Geometry check sheet. Reference: drawing and pictorial views, mm from the part's lowest x, y, z. Coordinates: 2 decimals unless noted, no trailing zeros. Write each loop counter-clockwise with the first axis right and the second up, starting at its lowest first coordinate (ties: lowest second). Pieces come first, ordered by that corner, then holes. Notation, with made-up numbers: (20.25, 89.5) - (72.25, 89.5) arc R24 ccw to (72.25, 103.5) - close; hole circle Ø1 at (8, 87). An arc over 180 degrees is marked (long way). Answer as a JSON object with one key per item and string values. Group by question number.
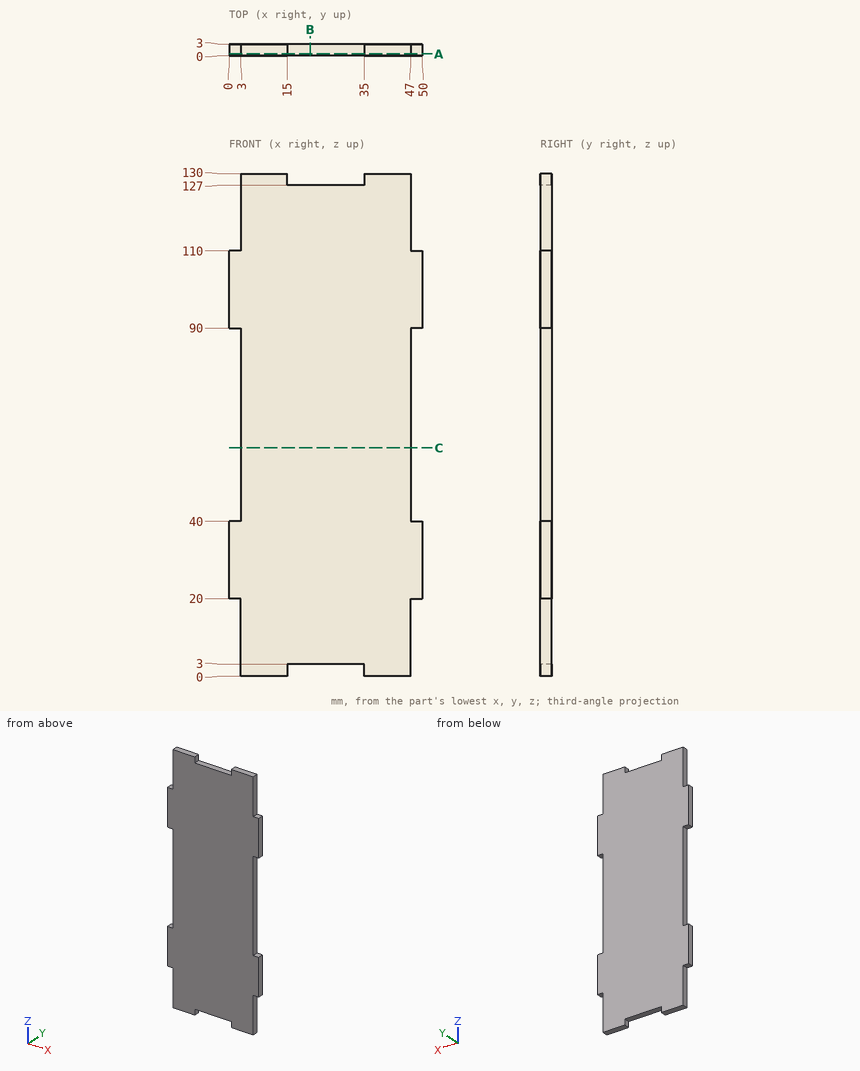
(1) Section check A-A (y = 0.45). Record the cut outline in (x, z).
(2) Material ranges on L1, parallel to Z at x = 47.5, y = 0.1; L2, parallel to Z at x = 25.5, y = 0.65; L3, parallel to X at y = 2.7, z = 123, recorded low to high. Write a range as [from, to].
(3) Section check B-B (x = 21). Record the cut outline in (y, z), and give its area (3 significant figures).
(4) Gauge pin test, flat ends, axial feed: pin 1 (1.5 mm diameter, centred on x = 1.5, y = 1.5, fed in from -Z); pin 2 (1 mm diameter, centred on x = 30, y = 1, fed in from +Z); pin 3 (1 mm diameter, centred on x = 40, z = 46.5, fed in from -Y); pin 4 (1.5 mm diameter, centred on x = 48, y = 1.5, fed in from +Z). Record the tip position at first contact, or that the pin passes through.
(5) Section check C-C (z = 59). Record the cut outline in (x, y).
Conclusion:
{
 "1": {"outline": "(0, 20) - (3, 20) - (3, 0) - (15, 0) - (15, 3) - (35, 3) - (35, 0) - (47, 0) - (47, 20) - (50, 20) - (50, 40) - (47, 40) - (47, 90) - (50, 90) - (50, 110) - (47, 110) - (47, 130) - (35, 130) - (35, 127) - (15, 127) - (15, 130) - (3, 130) - (3, 110) - (0, 110) - (0, 90) - (3, 90) - (3, 40) - (0, 40) - close"},
 "2": {"L1": "z = [20, 40], [90, 110]", "L2": "z = [3, 127]", "L3": "x = [3, 47]"},
 "3": {"outline": "(0, 3) - (3, 3) - (3, 127) - (0, 127) - close", "area": "372 mm^2"},
 "4": {"pin 1": "stops at z = 20", "pin 2": "stops at z = 127", "pin 3": "stops at y = 0", "pin 4": "stops at z = 110"},
 "5": {"outline": "(3, 0) - (47, 0) - (47, 3) - (3, 3) - close"}
}
